```python
from build123d import *

# Parameters (mm, degrees)
F0_W      = 15
F0_H      = 15
F1_DEPTH  = 5
F2_R      = 4
F3_DEPTH  = 25
F4_R      = 3
F5_DEPTH  = 2.5
F10_R     = 2.5
F11_DEPTH = 7


with BuildPart() as f1:
    # F0 (on Front) → F1 (new body)
    with BuildSketch(Plane.XZ):
        with Locations((-2.477283068, 5.5355651764)):
            Rectangle(F0_W, F0_H)
    extrude(amount=F1_DEPTH)

    # F2 (on face) → F3 (cut)
    with BuildSketch(Plane.XZ.offset(5)):
        with Locations((-2.477283068, 5.5355651764)):
            Circle(F2_R)
    extrude(amount=-F3_DEPTH, mode=Mode.SUBTRACT)

    # F4 (on face) → F5 (join)
    with BuildSketch(Plane.YZ.offset(5.022716932)):
        with Locations((-2.5, 5.5355651764)):
            Circle(F4_R)
    extrude(amount=F5_DEPTH)

    # F10 (on face) → F11 (join)
    with BuildSketch(Plane.YZ.offset(7.522716932)):
        with Locations((-2.5, 5.5355651764)):
            Circle(F10_R)
    extrude(amount=F11_DEPTH)

    # F12: F1 across plane


with BuildPart() as f1_1:
    add(f1.part)
    add(f1.part.mirror(Plane(origin=(-2.477283068, 0, 13.0355651764), x_dir=(0, -1, 0), z_dir=(-1, 0, 0))))


solid = f1_1.part
```
Geometry check sheet. Reference: the model listing, model coordinates, mm. A direction names the side the tool comes from. Round coordinates to 2 decimals unless told otherwise and drop trailing zeros. Loops run counter-clockwise (first coordinate to the right, second up) from the corner with the lowest first, then second, coordinate; pieces in that order, holes last. Notation, with made-up numbers: (-31.5, 26.25) - (17.5, 26.25) arc R21 ccw to (17.5, 53.25) - close; hole circle Ø5 at (57, 79.5). An arc over 180 degrees is marked (long way). Use a Markdown table: item, result.
Q1. Cross-section at B-B on z = 6.5. Record the cut outline in (x, y).
Solutions:
| item | result |
|---|---|
| outline | (-19.48, -4.81) - (-12.48, -4.81) - (-12.48, -5.34) - (-9.98, -5.34) - (-9.98, -5) - (-6.36, -5) - (-6.36, 0) - (-9.98, 0) - (-9.98, 0.34) - (-12.48, 0.34) - (-12.48, -0.19) - (-19.48, -0.19) - close; (1.4, -5) - (5.02, -5) - (5.02, -5.34) - (7.52, -5.34) - (7.52, -4.81) - (14.52, -4.81) - (14.52, -0.19) - (7.52, -0.19) - (7.52, 0.34) - (5.02, 0.34) - (5.02, 0) - (1.4, 0) - close |
Q2. Go/stop test with flat-tipped pins: P1, Ø1.5, axis at y = -2.5, z = 11.5, coming from the +X side; P2, Ø1, axis at x = 10, y = -2, coming from the -Z side; P3, Ø7.5, axis at x = -4, z = 7, coming from the +Y side. Record where each tip stops, or that it passes through.
Solutions:
| item | result |
|---|---|
| P1 | stops at x = 5.02 |
| P2 | stops at z = 3.04 |
| P3 | stops at y = 0 |
Q3. Cross-section at C-C on x = 4.5. Record the cut outline in (y, z).
Solutions:
| item | result |
|---|---|
| outline | (-5, -1.96) - (0, -1.96) - (0, 13.04) - (-5, 13.04) - close |
Q4. Access from +Z, -Z, +X, -X, +Y, -Y to the whole of each face (thin tool, end or side, straight path). Record for faces 1 (the flat face through (1, -5, 9)), 2 (the flat face through (1, 0, 9)), 3 (the cylindrical face through (-11.21, -2.89, 8.51)).
Solutions:
| item | result |
|---|---|
| face 1 | +Z, -Z, -Y |
| face 2 | +Z, -Z, +Y |
| face 3 | -X |
Q5. Cross-section at D-D on z = -0.5. Record the cut outline in (x, y), plus the area to 3 significant figures.
Solutions:
| item | result |
|---|---|
| outline | (-9.98, -5) - (5.02, -5) - (5.02, 0) - (-9.98, 0) - close |
| area | 75.0 mm2 |
Q6. Draft check along X on faces 4 (the cylindrical face through (-3.34, -2.54, 1.63)), 5 (the flat face through (5.023, -2, 0)), 6 (the flat face through (-9.977, -2, 0)), 7 (the cylindrical face through (-15.928, -3.042, 3.095)). Enter one of: released by +X, released by -X, zero draft, split by the parting line, or undercut.
Solutions:
| item | result |
|---|---|
| face 4 | undercut |
| face 5 | released by +X |
| face 6 | released by -X |
| face 7 | zero draft |
Q7. Cross-section at A-A on y = -2.5. Record the cut outline in (x, z).
Solutions:
| item | result |
|---|---|
| outline | (-19.48, 3.04) - (-12.48, 3.04) - (-12.48, 2.54) - (-9.98, 2.54) - (-9.98, -1.96) - (5.02, -1.96) - (5.02, 2.54) - (7.52, 2.54) - (7.52, 3.04) - (14.52, 3.04) - (14.52, 8.04) - (7.52, 8.04) - (7.52, 8.54) - (5.02, 8.54) - (5.02, 13.04) - (-9.98, 13.04) - (-9.98, 8.54) - (-12.48, 8.54) - (-12.48, 8.04) - (-19.48, 8.04) - close; hole circle Ø8 at (-2.48, 5.54) |
Q8. Material ranges on line 1 (X direction, y = -4.25, z = 10); line 2 (Y direction, x = -7, z = 6.75); line 3 (Z direction, x = 0, y = -3.8), recorded low to high.
Solutions:
| item | result |
|---|---|
| line 1 | x = -9.98 to 5.02 |
| line 2 | y = -5 to 0 |
| line 3 | z = -1.96 to 2.4, 8.68 to 13.04 |
